from build123d import *

# Parameters (mm, degrees)
CYLINDER002_R     = 1.5
CYLINDER002_DEPTH = 2
CYLINDER003_R     = 1.5
CYLINDER003_DEPTH = 2
CYLINDER004_R     = 1.5
CYLINDER004_DEPTH = 2
CYLINDER001_R     = 1.5
CYLINDER001_DEPTH = 2
CYLINDER_R        = 1.5
CYLINDER_DEPTH    = 2
BOX_W             = 31
BOX_H             = 7
BOX_DEPTH         = 2


with BuildPart() as cylinder002:
    # Cylinder002 → Cylinder002 (new body)
    with BuildSketch(Plane(origin=(15.5, 3.5, 0), x_dir=(1, 0, 0), z_dir=(0, 0, 1))):
        Circle(CYLINDER002_R)
    extrude(amount=CYLINDER002_DEPTH)


with BuildPart() as cylinder003:
    # Cylinder003 → Cylinder003 (new body)
    with BuildSketch(Plane(origin=(21.5, 3.5, 0), x_dir=(1, 0, 0), z_dir=(0, 0, 1))):
        Circle(CYLINDER003_R)
    extrude(amount=CYLINDER003_DEPTH)


with BuildPart() as cylinder004:
    # Cylinder004 → Cylinder004 (new body)
    with BuildSketch(Plane(origin=(9.5, 3.5, 0), x_dir=(1, 0, 0), z_dir=(0, 0, 1))):
        Circle(CYLINDER004_R)
    extrude(amount=CYLINDER004_DEPTH)


with BuildPart() as cylinder001:
    # Cylinder001 → Cylinder001 (new body)
    with BuildSketch(Plane(origin=(27.5, 3.5, 0), x_dir=(1, 0, 0), z_dir=(0, 0, 1))):
        Circle(CYLINDER001_R)
    extrude(amount=CYLINDER001_DEPTH)


with BuildPart() as cylinder:
    # Cylinder → Cylinder (new body)
    with BuildSketch(Plane(origin=(3.5, 3.5, 0), x_dir=(1, 0, 0), z_dir=(0, 0, 1))):
        Circle(CYLINDER_R)
    extrude(amount=CYLINDER_DEPTH)


with BuildPart() as cut004:
    # Box → Box (new body)
    with BuildSketch(Plane.XY):
        with Locations((15.5, 3.5)):
            Rectangle(BOX_W, BOX_H)
    extrude(amount=BOX_DEPTH)

    # Cut: cut Cylinder
    add(cylinder.part, mode=Mode.SUBTRACT)

    # Cut001: cut Cylinder001
    add(cylinder001.part, mode=Mode.SUBTRACT)

    # Cut002: cut Cylinder004
    add(cylinder004.part, mode=Mode.SUBTRACT)

    # Cut003: cut Cylinder003
    add(cylinder003.part, mode=Mode.SUBTRACT)

    # Cut004: cut Cylinder002
    add(cylinder002.part, mode=Mode.SUBTRACT)


solid = cut004.part
Verification items for the finished model (mm, model axes). Give positions to 0.01 mm unless a question says otherwise; leave off trailing zeros. Write each loop counter-clockwise with the first axis right and the second up, starting at its lowest first coordinate (ties: lowest second). Pieces come first, ordered by that corner, then holes. Notation, with made-up numbers: M -33,-35 L -6,-35 A30 cw -6,3 Z; hole C -20.75,-30 d6. An arc over 180 degrees is marked long. Use CSV: the item, a comma, the result in double quotes.
1) Material ranges on line 1 along Y through (x, z) = (27.5, 1.8); line 2 along X through (y, z) = (2.25, 0.15); line 3 along X through (y, z) = (3, 1.5), recorded low to high.
Final values:
line 1,"0 to 2, 5 to 7"
line 2,"0 to 2.67, 4.33 to 8.67, 10.33 to 14.67, 16.33 to 20.67, 22.33 to 26.67, 28.33 to 31"
line 3,"0 to 2.09, 4.91 to 8.09, 10.91 to 14.09, 16.91 to 20.09, 22.91 to 26.09, 28.91 to 31"
2) Release check for a two-part mould opening along X. For faces 1 (the face through (0, 3, 1)), 2 (the face through (26, 3.57, 0.99)), 3 (the face through (15, 6, 0)) record: released by +X, released by -X, zero draft, split by the parting line, or undercut.
Final values:
face 1,"released by -X"
face 2,"undercut"
face 3,"zero draft"
3) Cross-section at D-D (x = 8.5). Enter the section's corners in (y, z).
Final values:
outline,"M 0,0 L 2.38,0 L 2.38,2 L 0,2 Z; M 4.62,0 L 7,0 L 7,2 L 4.62,2 Z"
4) Cross-section at C-C (z = 1.35). Enter the section's corners in (x, y).
Final values:
outline,"M 0,0 L 31,0 L 31,7 L 0,7 Z; hole C 3.5,3.5 d3; hole C 9.5,3.5 d3; hole C 15.5,3.5 d3; hole C 21.5,3.5 d3; hole C 27.5,3.5 d3"
5) Go/stop test with flat-tipped pins: pin 1 Ø1.8 at (x, y) = (21.5, 3.5) entering from -Z; pin 2 Ø4 at (x, y) = (9.5, 3.5) entering from +Z. Record where each tip stops, or that it passes through.
Final values:
pin 1,"through"
pin 2,"z = 2"
6) Cross-section at B-B (x = 3.5). Enter the section's corners in (y, z), plus the area to 3 significant figures.
Final values:
outline,"M 0,0 L 2,0 L 2,2 L 0,2 Z; M 5,0 L 7,0 L 7,2 L 5,2 Z"
area,"8.00 mm²"
7) Cross-section at A-A (y = 3.5). Enter the section's corners in (x, z), plus the area to 3 significant figures.
Final values:
outline,"M 0,0 L 2,0 L 2,2 L 0,2 Z; M 5,0 L 8,0 L 8,2 L 5,2 Z; M 11,0 L 14,0 L 14,2 L 11,2 Z; M 17,0 L 20,0 L 20,2 L 17,2 Z; M 23,0 L 26,0 L 26,2 L 23,2 Z; M 29,0 L 31,0 L 31,2 L 29,2 Z"
area,"32.0 mm²"
